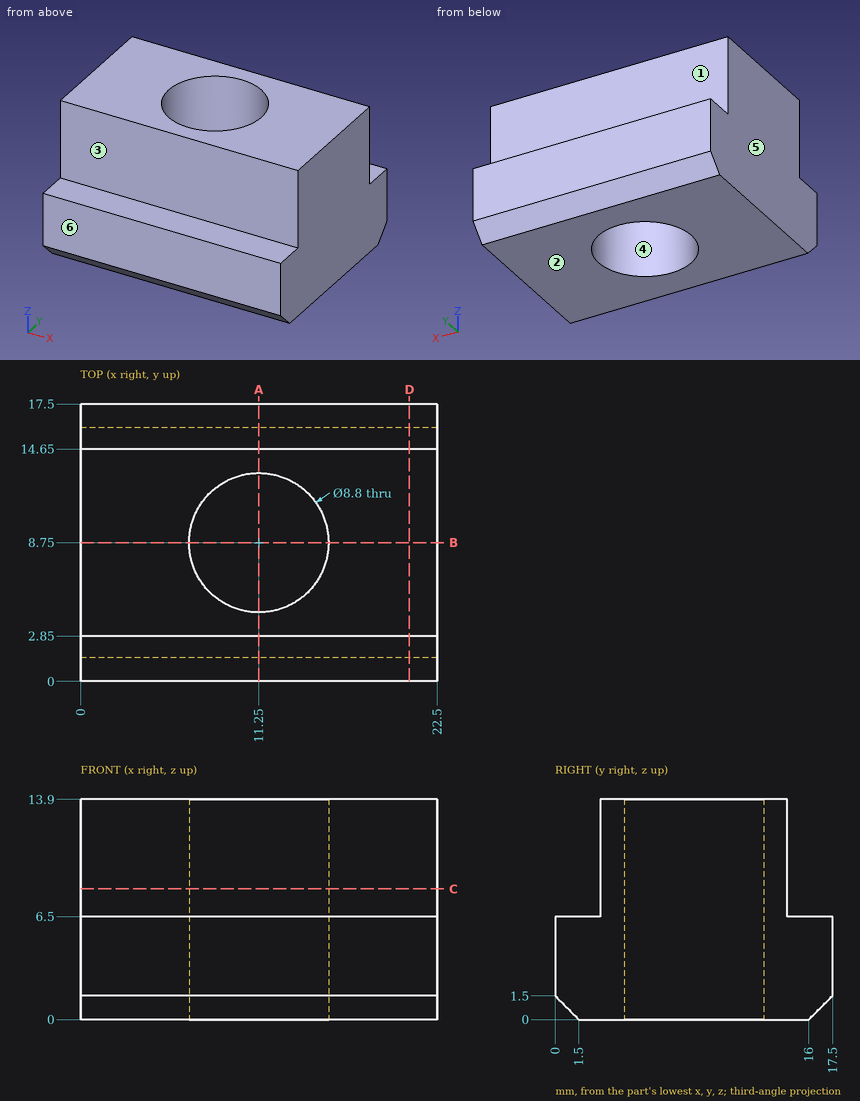
Study the drawing (mm; zero at the part's minimum x, y, z) and answer. A direction names the side the tool comes from. Coordinates: 2 decimals unless noted, no trailing zeros. Order: outer loops, then holes, each group sorted by start corner. A loop starts at its lowest first (then second) coordinate and runs counter-clockwise, first axis right, second up. Notation, with made-up numbers: M 49.5,20.5 L 78.5,20.5 A8 cw 78.5,34.5 Z; hole C 88,45 d10. An arc over 180 degrees is marked long. Answer as a JSON object with one key per item and string values. Group by question number.
1. Straight lines are drawn through the part: line 1 (X direction, y = 8.5, z = 8.5); line 2 (Y direction, x = 11.25, z = 4); line 3 (Y direction, x = 21.5, z = 12.5). For each, find the intervals that lie inside material, in ascending order.
2. Flat-ended cylindrical pins translate along their axes: P1, Ø8, axis at x = 6.5, z = 11.5, coming from the -Y side; P2, Ø1.4, axis at x = 16.5, y = 1, coming from the +Z side; P3, Ø1, axis at x = 6.5, z = 8, coming from the +Y side. Find the tip coordinate at first contact, or state that the pin passes through.
3. Section A-A on x = 11.25 is taken. Write down the section's boundary in (y, z).
4. A tool of negligible diameter and unlimited length cuts with its end or side. For the marked faces 1, 2 and 3, from which of +Z, -Z, +X, -X, +Y, -Y can it reach the whole face along a straight path? Write none if from no direction.
5. Section B-B on y = 8.75 is taken. Write down the section's boundary in (x, z), then the cut area to 3 significant figures.
6. Determine the mould class of the marked faces 4, 5 and 6 for opening direction X: released by +X, released by -X, zero draft, split by the parting line, or undercut.
7. Section D-D on x = 20.75 is taken. Write down the section's boundary in (y, z).
8. Section C-C on z = 8.25 is taken. Write down the section's boundary in (x, y), then the cut area to 3 significant figures.
Values follow:
{
 "1": {"line 1": "0 to 6.86, 15.64 to 22.5", "line 2": "0 to 4.35, 13.15 to 17.5", "line 3": "2.85 to 14.65"},
 "2": {"P1": "y = 2.85", "P2": "z = 6.5", "P3": "y = 14.65"},
 "3": {"outline": "M 0,1.5 L 1.5,0 L 4.35,0 L 4.35,13.9 L 2.85,13.9 L 2.85,6.5 L 0,6.5 Z; M 13.15,0 L 16,0 L 17.5,1.5 L 17.5,6.5 L 14.65,6.5 L 14.65,13.9 L 13.15,13.9 Z"},
 "4": {"face 1": "+Z, +X, -X, +Y", "face 2": "-Z, +X, -X, +Y, -Y", "face 3": "+Z, +X, -X, -Y"},
 "5": {"outline": "M 0,0 L 6.85,0 L 6.85,13.9 L 0,13.9 Z; M 15.65,0 L 22.5,0 L 22.5,13.9 L 15.65,13.9 Z", "area": "190 mm2"},
 "6": {"face 4": "undercut", "face 5": "released by -X", "face 6": "zero draft"},
 "7": {"outline": "M 0,1.5 L 1.5,0 L 16,0 L 17.5,1.5 L 17.5,6.5 L 14.65,6.5 L 14.65,13.9 L 2.85,13.9 L 2.85,6.5 L 0,6.5 Z"},
 "8": {"outline": "M 0,2.85 L 22.5,2.85 L 22.5,14.65 L 0,14.65 Z; hole C 11.25,8.75 d8.8", "area": "205 mm2"}
}
